from build123d import *

# Parameters (mm, degrees)
ESQUISSE1_W             = 120
ESQUISSE1_H             = 160
BOSS_EXTRU_1_DEPTH      = 40
CONG_1_R                = 10
CONG_2_R                = 10
ESQUISSE2_W             = 110
ESQUISSE2_H             = 150
ENL_V_MAT_EXTRU_1_DEPTH = 35
CONG_3_R                = 10
ESQUISSE3_R             = 3
ENL_V_MAT_EXTRU_2_DEPTH = 35
ESQUISSE4_R             = 2.5
BOSS_EXTRU_2_DEPTH      = 2.5
CONG_4_R                = 2.5
ESQUISSE5_W             = 11
ESQUISSE5_H             = 52
ESQUISSE5_W_2           = 52
ESQUISSE5_H_2           = 11
ENL_V_MAT_EXTRU_3_DEPTH = 2
ESQUISSE6_W             = 26
ESQUISSE6_H             = 22
ENL_V_MAT_EXTRU_4_DEPTH = 2
ESQUISSE7_W             = 26
ESQUISSE7_H             = 22
ENL_V_MAT_EXTRU_5_DEPTH = 2
ESQUISSE8_W             = 27
ESQUISSE8_H             = 22
ENL_V_MAT_EXTRU_6_DEPTH = 5
ESQUISSE9_R             = 1
ENL_V_MAT_EXTRU_7_DEPTH = 4
ESQUISSE10_W            = 11
ESQUISSE10_H            = 6
ENL_V_MAT_EXTRU_8_DEPTH = 201.062490237
ESQUISSE11_W            = 11
ESQUISSE11_H            = 10
ENL_V_MAT_EXTRU_9_DEPTH = 3


with BuildPart() as part:
    # Esquisse1 → Boss.-Extru.1 (new body)
    with BuildSketch(Plane(origin=(0, 0, 0), x_dir=(1, 0, 0), z_dir=(0, 1, 0))):
        with Locations((60, 80)):
            Rectangle(ESQUISSE1_W, ESQUISSE1_H)
    extrude(amount=BOSS_EXTRU_1_DEPTH)

    # Congé1
    cong_1_edges = [part.edges().sort_by_distance(p)[0] for p in [
        (60, 0, -160),
    ]]
    fillet(cong_1_edges, radius=CONG_1_R)

    # Congé2
    cong_2_edges = [part.edges().sort_by_distance(p)[0] for p in [
        (120, 2.928932188, -157.071067812),
        (120, 0, -75),
        (120, 25, -160),
    ]]
    fillet(cong_2_edges, radius=CONG_2_R)

    # Esquisse2 → Enlèv. mat.-Extru.1 (cut)
    with BuildSketch(Plane(origin=(0, 40, 0), x_dir=(1, 0, 0), z_dir=(0, 1, 0))):
        with Locations((55, 75)):
            Rectangle(ESQUISSE2_W, ESQUISSE2_H)
    extrude(amount=-ENL_V_MAT_EXTRU_1_DEPTH, mode=Mode.SUBTRACT)

    # Congé3
    cong_3_edges = [part.edges().sort_by_distance(p)[0] for p in [
        (110, 22.5, -150),
    ]]
    fillet(cong_3_edges, radius=CONG_3_R)

    # Esquisse3 → Enlèv. mat.-Extru.2 (cut)
    with BuildSketch(Plane(origin=(0, 40, 0), x_dir=(1, 0, 0), z_dir=(0, 1, 0))):
        with Locations(Location((112, 152, 0), (0, 0, 270))):
            Circle(ESQUISSE3_R)
    extrude(amount=-ENL_V_MAT_EXTRU_2_DEPTH, mode=Mode.SUBTRACT)

    # Esquisse4 → Boss.-Extru.2 (add)
    with BuildSketch(Plane.XZ):
        with Locations(Location((90, -130, 0), (0, 0, 270))):
            Circle(ESQUISSE4_R)
    extrude(amount=BOSS_EXTRU_2_DEPTH)

    # Congé4
    cong_4_edges = [part.edges().sort_by_distance(p)[0] for p in [
        (90, -2.5, -127.5),
    ]]
    fillet(cong_4_edges, radius=CONG_4_R - 0.0001)  # a hair under: the kernel refuses the full size

    # Esquisse5 → Enlèv. mat.-Extru.3 (cut)
    with BuildSketch(Plane(origin=(0, 5, 0), x_dir=(1, 0, 0), z_dir=(0, 1, 0))):
        with Locations((5.5, 75)):
            Rectangle(ESQUISSE5_W, ESQUISSE5_H)
        with Locations((55, 5.5)):
            Rectangle(ESQUISSE5_W_2, ESQUISSE5_H_2)
    extrude(amount=-ENL_V_MAT_EXTRU_3_DEPTH, mode=Mode.SUBTRACT)

    # Esquisse6 → Enlèv. mat.-Extru.4 (cut)
    with BuildSketch(Plane.XY.offset(-150)):
        with Locations((13, 22.5)):
            Rectangle(ESQUISSE6_W, ESQUISSE6_H)
    extrude(amount=-ENL_V_MAT_EXTRU_4_DEPTH, mode=Mode.SUBTRACT)

    # Esquisse7 → Enlèv. mat.-Extru.5 (cut)
    with BuildSketch(Plane.ZY.offset(-110)):
        with Locations((-13, 22.5)):
            Rectangle(ESQUISSE7_W, ESQUISSE7_H)
    extrude(amount=-ENL_V_MAT_EXTRU_5_DEPTH, mode=Mode.SUBTRACT)

    # Esquisse8 → Enlèv. mat.-Extru.6 (cut)
    with BuildSketch(Plane.XY.offset(-150)):
        with Locations((46.5, 22)):
            Rectangle(ESQUISSE8_W, ESQUISSE8_H)
    extrude(amount=-ENL_V_MAT_EXTRU_6_DEPTH, mode=Mode.SUBTRACT)

    # Esquisse9 → Enlèv. mat.-Extru.7 (cut)
    with BuildSketch(Plane.XY.offset(-155)):
        with Locations((56.75, 22)):
            Circle(ESQUISSE9_R)
        with Locations((36.25, 22)):
            Circle(ESQUISSE9_R)
    extrude(amount=-ENL_V_MAT_EXTRU_7_DEPTH, mode=Mode.SUBTRACT)

    # Esquisse10 → Enlèv. mat.-Extru.8 (cut, through all)
    with BuildSketch(Plane.XY.offset(-155)):
        with Locations((46.5, 26)):
            Rectangle(ESQUISSE10_W, ESQUISSE10_H)
    extrude(amount=-ENL_V_MAT_EXTRU_8_DEPTH, mode=Mode.SUBTRACT)

    # Esquisse11 → Enlèv. mat.-Extru.9 (cut)
    with BuildSketch(Plane.XY.offset(-155)):
        with Locations((46.5, 18)):
            Rectangle(ESQUISSE11_W, ESQUISSE11_H)
    extrude(amount=-ENL_V_MAT_EXTRU_9_DEPTH, mode=Mode.SUBTRACT)


solid = part.part
Can you work these out from the model? Positions are in its coordinate system, mm. A direction names the side the tool comes from. Give positions to 0.01 mm unless a question says otherwise; leave off trailing zeros. Write each loop counter-clockwise with the first axis right and the second up, starting at its lowest first coordinate (ties: lowest second). Pieces come first, ordered by that corner, then holes. Notation, with made-up numbers: (38.5, 72.25) -> (90.5, 72.25) arc R22 cw to (90.5, 107.25) -> close; hole circle Ø1 at (15.5, -20.5). An arc over 180 degrees is marked (long way). Answer as a JSON object with one key per item and string values. Group by question number.
Item 1: Please list where these lines run through material, in increasing order: line 1 (Z direction, x = 66, y = 17.5); line 2 (X direction, y = 34, z = -137); line 3 (Y direction, x = 36, z = -156). Write a range as [from, to].
Item 2: Suppose I cut it at C-C (x = 63.5). Please give me the cut outline in (y, z).
Item 3: We'd pull the mould along Y, two halves only. Please class faces 6 (the face through (46, 33, -152)), 7 (the face through (55.77, 3.01, -157.15)), 8 (the face through (106.99, 22.26, -147.15)), 9 (the face through (46, 29, -157)): +Y half, -Y half, draft (parallel to the pull), parting line (faces both ways), or undercut.
Item 4: Suppose I cut it at D-D (z = -92). Please give me the cut outline in (x, y), plus the area to 3 significant figures.
Item 5: I'm going to push flat-ended pins straight in: P1, Ø6, axis at x = 34, z = -135.5, coming from the +Y side; P2, Ø1.8, axis at x = 36.25, y = 22, coming from the +Z side; P3, Ø2.5, axis at y = 24, z = -153.5, coming from the +X side; P4, Ø2, axis at y = 4, z = -8, coming from the -X side. Where does each tip first touch, or does it pass through?
Item 6: Suppose I cut it at A-A (z = -30). Please give me the cut outline in (x, y).
Item 7: Suppose I cut it at B-B (y = 36). Please give me the cut outline in (x, z), plus the area to 3 significant figures.
Item 8: For faces 1 (the face through (13, 23, -152)), 2 (the face through (113, 40, -110)), 3 (the face through (33, 22, -152)), 4 (the face through (54, 5, -76)), 5 (the face through (120, 25, -74)), which set-ups out of +Z, -Z, +X, -X, +Y, -Y let a thin tool reach every point of the face, with its end or its side?
Findings:
{
 "1": {"line 1": "z = [-160, -150]", "line 2": "x = [110, 120]", "line 3": "y = [2, 21.03], [22.97, 40]"},
 "2": {"outline": "(0, -150) arc R10 ccw to (10, -160) -> (40, -160) -> (40, -150) -> (5, -150) -> (5, -11) -> (3, -11) -> (3, 0) -> (0, 0) -> close"},
 "3": {"face 6": "undercut", "face 7": "-Y half", "face 8": "draft", "face 9": "undercut"},
 "4": {"outline": "(0, 0) -> (110, 0) arc R10 ccw to (120, 10) -> (120, 40) -> (110, 40) -> (110, 5) -> (11, 5) -> (11, 3) -> (0, 3) -> close", "area": "907 mm²"},
 "5": {"P1": "stops at y = 5", "P2": "stops at z = -159", "P3": "stops at x = 119.74", "P4": "stops at x = 0"},
 "6": {"outline": "(0, 0) -> (110, 0) arc R10 ccw to (120, 10) -> (120, 40) -> (110, 40) -> (110, 5) -> (0, 5) -> close"},
 "7": {"outline": "(0, -160) -> (110, -160) arc R10 ccw to (120, -150) -> (120, 0) -> (110, 0) -> (110, -140) arc R10 cw to (100, -150) -> (0, -150) -> close; hole circle Ø6 at (112, -152)", "area": "2,670 mm²"},
 "8": {"face 1": "+Z, -X", "face 2": "+Z, -Z, +X, -X, +Y", "face 3": "+Z", "face 4": "+Z, -X, +Y", "face 5": "+Z, -Z, +X, +Y, -Y"}
}
